```python
from build123d import *

# Parameters (mm, degrees)
CROQUIS1_R              = 10.45
CROQUIS1_R_2            = 4.25
SALIENTE_EXTRUIR1_DEPTH = 3.6
CROQUIS1_3_R            = 4.25
CROQUIS1_3_R_2          = 3
SALIENTE_EXTRUIR2_DEPTH = 6
CORTAR_EXTRUIR1_REACH   = 17.95
CROQUIS3_R              = 1
SALIENTE_EXTRUIR3_START = -1
CROQUIS4_R              = 3
SALIENTE_EXTRUIR3_DEPTH = 1
CROQUIS5_R              = 1.5
CORTAR_EXTRUIR2_DEPTH   = 1


with BuildPart() as part:
    # Croquis1 → Saliente-Extruir1 (new body)
    with BuildSketch(Plane(origin=(0, 0, 0), x_dir=(1, 0, 0), z_dir=(0, 1, 0))):
        with Locations(Location((0, 0, 0), (0, 0, 270))):
            Circle(CROQUIS1_R)
        with Locations(Location((0, 0, 0), (0, 0, 270))):
            Circle(CROQUIS1_R_2, mode=Mode.SUBTRACT)
    extrude(amount=-SALIENTE_EXTRUIR1_DEPTH)

    # Croquis1<3> → Saliente-Extruir2 (add)
    with BuildSketch(Plane(origin=(0, 0, 0), x_dir=(1, 0, 0), z_dir=(0, 1, 0))):
        with Locations(Location((0, 0, 0), (0, 0, 270))):
            Circle(CROQUIS1_3_R)
        with Locations(Location((0, 0, 0), (0, 0, 270))):
            Circle(CROQUIS1_3_R_2, mode=Mode.SUBTRACT)
    extrude(amount=-SALIENTE_EXTRUIR2_DEPTH)

    # Croquis3 → Cortar-Extruir1 (cut, up to next)
    with BuildSketch(Plane(origin=(0, 0, 0), x_dir=(1, 0, 0), z_dir=(0, 1, 0)), mode=Mode.PRIVATE) as cortar_extruir1_sk1:
        with Locations(Location((7, 0, 0), (0, 0, 270))):
            Circle(CROQUIS3_R)
    cortar_extruir1_tool1 = extrude(cortar_extruir1_sk1.sketch, amount=-CORTAR_EXTRUIR1_REACH, mode=Mode.PRIVATE) & part.part
    # Croquis3 → Cortar-Extruir1 (cut, up to next)
    with BuildSketch(Plane(origin=(0, 0, 0), x_dir=(1, 0, 0), z_dir=(0, 1, 0)), mode=Mode.PRIVATE) as cortar_extruir1_sk2:
        with Locations(Location((-7, 0, 0), (0, 0, 270))):
            Circle(CROQUIS3_R)
    cortar_extruir1_tool2 = extrude(cortar_extruir1_sk2.sketch, amount=-CORTAR_EXTRUIR1_REACH, mode=Mode.PRIVATE) & part.part
    add(cortar_extruir1_tool1.solids().sort_by_distance((7, 0, 0))[0], mode=Mode.SUBTRACT)
    add(cortar_extruir1_tool2.solids().sort_by_distance((-7, 0, 0))[0], mode=Mode.SUBTRACT)

    # Croquis4 → Saliente-Extruir3 (add)
    with BuildSketch(Plane(origin=(0, 0, 0), x_dir=(1, 0, 0), z_dir=(0, 1, 0)).offset(SALIENTE_EXTRUIR3_START)):
        with Locations(Location((0, 0, 0), (0, 0, 270))):
            Circle(CROQUIS4_R)
    extrude(amount=-SALIENTE_EXTRUIR3_DEPTH)

    # Croquis5 → Cortar-Extruir2 (cut)
    with BuildSketch(Plane(origin=(0, -1, 0), x_dir=(1, 0, 0), z_dir=(0, 1, 0))):
        with Locations(Location((0, 0, 0), (0, 0, 270))):
            Circle(CROQUIS5_R)
    extrude(amount=-CORTAR_EXTRUIR2_DEPTH, mode=Mode.SUBTRACT)


solid = part.part
```
Geometry check sheet. Reference: the model listing, model coordinates, mm. A direction names the side the tool comes from. Coordinates: 2 decimals unless noted, no trailing zeros. Order: outer loops, then holes, each group sorted by start corner. A loop starts at its lowest first (then second) coordinate and runs counter-clockwise, first axis right, second up. Notation, with made-up numbers: M 7.25,-39.5 L 65.25,-39.5 A21 cw 65.25,-35.5 Z; hole C 87,46 d5. An arc over 180 degrees is marked long. One line per question, with ' | ' between items. Start each with the question number.
Item 1: Cross-section at C-C on y = -1.7. Enter the section's corners in (x, z).
Item 2: Set-up check for faces 1 (the flat face through (0.1, -3.6, 4.5)), 2 (the cylindrical face through (0.9, -0.49, 2.86)), 3 (the flat face through (-1, -6, -3)): record each of +Z, -Z, +X, -X, +Y, -Y from which the full face is reachable in a straight line by a thin tool's end or side.
Item 3: Draft check along X on faces 4 (the cylindrical face through (8, -2, 0)), 5 (the cylindrical face through (3.139, -1.775, 9.967)), 6 (the flat face through (2.5, 0, 2.2)). Enter one of: pulls with the +X half, pulls with the -X half, needs draft (parallel to the pull), parting line crosses it, or undercut.
Item 4: Gauge pin test, flat ends, axial feed: pin 1 (6.5 mm diameter, centred on x = -1, z = -1, fed in from -Y); pin 2 (1 mm diameter, centred on y = -4, z = -4.5, fed in from -X); pin 3 (3.5 mm diameter, centred on x = 0, z = 0, fed in from +Y); pin 4 (1.2 mm diameter, centred on x = 7, z = 0, fed in from -Y). Record the tip position at first contact, or that the pin passes through.
Item 5: Cross-section at A-A on z = 0. Enter the section's corners in (x, y).
Item 6: Cross-section at D-D on x = 0. Enter the section's corners in (y, z), then the cut area to 3 significant figures.
Item 7: Material ranges on L1, parallel to X at y = -0.45, z = 0; L2, parallel to X at y = -1.9, z = -0.5; L3, parallel to Y at x = 5.25, z = -4.25, recorded low to high. Write a range as [from, to].
Item 8: Cross-section at B-B on x = -7. Enter the section's corners in (y, z).
Findings:
1) outline: C 0,0 d20.9; hole C -7,0 d2; hole C 0,0 d3; hole C 7,0 d2
2) face 1: -Y | face 2: +Y | face 3: +Z, -Z, +X, -X, -Y
3) face 4: undercut | face 5: parting line crosses it | face 6: needs draft
4) pin 1: stops at y = -6 | pin 2: stops at x = -9.57 | pin 3: stops at y = -1 | pin 4: passes through
5) outline: M -10.45,-3.6 L -8,-3.6 L -8,0 L -10.45,0 Z; M -6,-3.6 L -4.25,-3.6 L -4.25,-6 L -3,-6 L -3,-2 L -1.5,-2 L -1.5,-1 L -3,-1 L -3,0 L -6,0 Z; M 1.5,-2 L 3,-2 L 3,-6 L 4.25,-6 L 4.25,-3.6 L 6,-3.6 L 6,0 L 3,0 L 3,-1 L 1.5,-1 Z; M 8,-3.6 L 10.45,-3.6 L 10.45,0 L 8,0 Z
6) outline: M -6,-4.25 L -3.6,-4.25 L -3.6,-10.45 L 0,-10.45 L 0,-3 L -1,-3 L -1,-1.5 L -2,-1.5 L -2,-3 L -6,-3 Z; M -6,3 L -2,3 L -2,1.5 L -1,1.5 L -1,3 L 0,3 L 0,10.45 L -3.6,10.45 L -3.6,4.25 L -6,4.25 Z | area: 62.6 mm²
7) L1: x = [-10.45, -8], [-6, -3], [3, 6], [8, 10.45] | L2: x = [-10.44, -7.87], [-6.13, -1.41], [1.41, 6.13], [7.87, 10.44] | L3: y = [-3.6, 0]
8) outline: M -3.6,-7.76 L 0,-7.76 L 0,-1 L -3.6,-1 Z; M -3.6,1 L 0,1 L 0,7.76 L -3.6,7.76 Z
